Job drawing, mm, ordinate dimensions from the low corner. One solid piece. Give positions to 0.01 mm unless a question says otherwise; leave off trailing zeros. Loops run counter-clockwise (first coordinate to the right, second up) from the corner with the lowest first, then second, coordinate; pieces in that order, holes last. Notation, with made-up numbers: M 41,24 L 95,24 A26 ccw 95,45 Z; hole C 77.5,10 d3. An arc over 180 degrees is marked long. Answer in a Markdown table with one row per item.
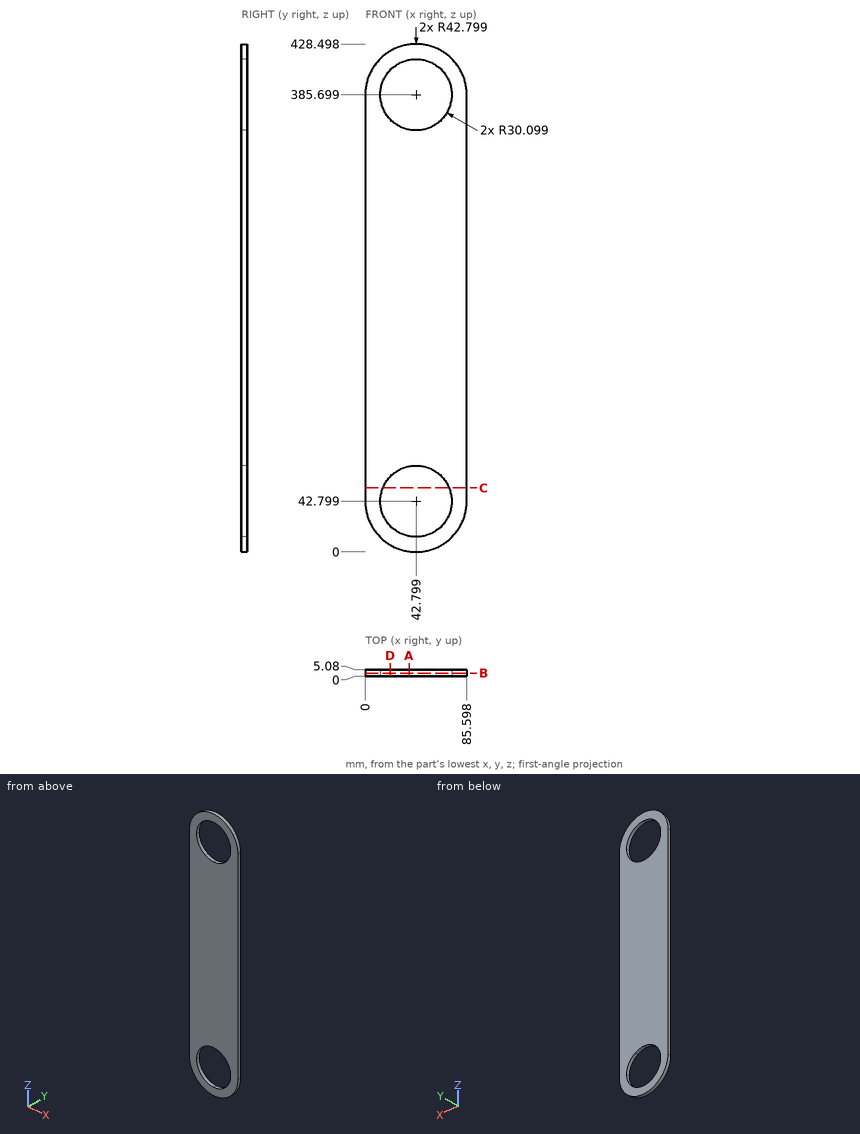
(1) Saw through at C-C (z = 54). Write the cut outline in (x, y), plus the area to 3 significant figures.
Recorded:
| item | result |
|---|---|
| outline | M 0,0 L 14.86,0 L 14.86,5.08 L 0,5.08 Z; M 70.74,0 L 85.6,0 L 85.6,5.08 L 70.74,5.08 Z |
| area | 151 mm^2 |
(2) Saw through at D-D (x = 21). Write the cut outline in (y, z), plus the area to 3 significant figures.
Recorded:
| item | result |
|---|---|
| outline | M 0,5.97 L 5.08,5.97 L 5.08,22.04 L 0,22.04 Z; M 0,63.55 L 5.08,63.55 L 5.08,364.94 L 0,364.94 Z; M 0,406.45 L 5.08,406.45 L 5.08,422.53 L 0,422.53 Z |
| area | 1,690 mm^2 |
(3) Saw through at B-B (y = 2.4). Write the cut outline in (x, z), plus the area to 3 significant figures.
Recorded:
| item | result |
|---|---|
| outline | M 0,42.8 A42.8 ccw 85.6,42.8 L 85.6,385.7 A42.8 ccw 0,385.7 Z; hole C 42.8,42.8 d60.2; hole C 42.8,385.7 d60.2 |
| area | 29,400 mm^2 |
(4) Pin check, flat tips, straight feed: pin 1 Ø1 at (x, y) = (42.5, 4.5) entering from +Z; pin 2 Ø8 at (x, z) = (70.5, 104.5) entering from -Y; pin 3 Ø3 at (x, y) = (69, 2.5) entering from -Z; pin 4 Ø1 at (x, y) = (50.5, 2.5) entering from -Z. Stop position of each tip, or through.
Recorded:
| item | result |
|---|---|
| pin 1 | stops at z = 428.5 |
| pin 2 | stops at y = 0 |
| pin 3 | stops at z = 7.85 |
| pin 4 | stops at z = 0.61 |
(5) Saw through at A-A (x = 37). Write the cut outline in (y, z).
Recorded:
| item | result |
|---|---|
| outline | M 0,0.39 L 5.08,0.39 L 5.08,13.26 L 0,13.26 Z; M 0,72.33 L 5.08,72.33 L 5.08,356.16 L 0,356.16 Z; M 0,415.23 L 5.08,415.23 L 5.08,428.1 L 0,428.1 Z |
(6) Drill centre lines: line 1 along Z through (x, y) = (43.5, 2.75); line 2 along Z through (x, y) = (28.5, 4.8); line 3 along X through (y, z) = (1.85, 48). Where is each one in solid material? Low to high.
Recorded:
| item | result |
|---|---|
| line 1 | z = 0.01 to 12.71, 72.89 to 355.61, 415.79 to 428.49 |
| line 2 | z = 2.46 to 16.31, 69.28 to 359.21, 412.18 to 426.04 |
| line 3 | x = 0 to 13.15, 72.45 to 85.6 |
